```python
from build123d import *

# Parameters (mm, degrees)
SKETCH2_W                   = 29
SKETCH2_H                   = 27.475014389
BOSS_EXTRUDE1_DEPTH         = 2
SKETCH7_W                   = 45
SKETCH7_H                   = 2
BOSS_EXTRUDE2_DEPTH         = 15
TAP_DRILL_FOR_M2X0_4_TAP1_D = 1.6
TAP_DRILL_FOR_M2X0_4_TAP2_D = 1.6


with BuildPart() as part:
    # Sketch2 → Boss-Extrude1 (new body)
    with BuildSketch(Plane(origin=(0, 0, 0), x_dir=(1, 0, 0), z_dir=(0, 1, 0))):
        with Locations((-24.397211382, -13.737507195)):
            Rectangle(SKETCH2_W, SKETCH2_H)
    extrude(amount=BOSS_EXTRUDE1_DEPTH)

    # Sketch7 → Boss-Extrude2 (add)
    with BuildSketch(Plane(origin=(0, 0, 0), x_dir=(-1, 0, 0), z_dir=(0, -1, 0))):
        with Locations((24.397211382, 0.886680676)):
            Rectangle(SKETCH7_W, SKETCH7_H)
    extrude(amount=-BOSS_EXTRUDE2_DEPTH)

    # Tap Drill for M2x0.4 Tap1 (through all)
    with Locations(Plane.XY.offset(0.113319324)):
        with Locations((-42.897211382, 4)):
            Hole(TAP_DRILL_FOR_M2X0_4_TAP1_D / 2)

    # Tap Drill for M2x0.4 Tap2 (through all)
    with Locations(Plane.XY.offset(0.113319324)):
        with Locations((-5.897211382, 4)):
            Hole(TAP_DRILL_FOR_M2X0_4_TAP2_D / 2)


solid = part.part
```
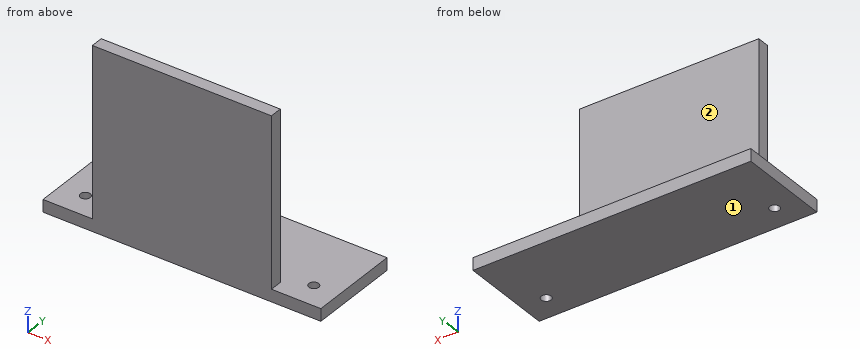
Model file for the job. Use its own axes, mm. Face numbers are marked on the shaded views. A direction names the side the tool comes from. Coordinates: 2 decimals unless noted, no trailing zeros. Loops run counter-clockwise (first coordinate to the right, second up) from the corner with the lowest first, then second, coordinate; pieces in that order, holes last. Notation, with made-up numbers: (16, 83.5) -> (65, 83.5) arc R28 ccw to (65, 120.5) -> close; hole circle Ø6 at (22.5, -17.75). An arc over 180 degrees is marked (long way). Answer as a JSON object with one key per item and string values.
Q1. Flat gauge pins, fed straight in: P1, Ø1, axis at x = -42.9, y = 4, coming from the +Z side; P2, Ø1.6, axis at y = 0.5, z = 7.5, coming from the +X side; P3, Ø4, axis at x = -38.5, z = 13.5, coming from the +Y side; P4, Ø7.5, axis at x = -26, y = 6, coming from the +Z side. Where does each tip first touch, or does it go through?
Report:
{"P1": "passes through", "P2": "stops at x = -9.9", "P3": "stops at y = 2", "P4": "stops at z = 0.11"}
Q2. Cut at A-A (y = 4). List the corners of the cut face in (x, z), and give its area (3 significant figures).
Report:
{"outline": "(-46.9, -1.89) -> (-43.7, -1.89) -> (-43.7, 0.11) -> (-46.9, 0.11) -> close; (-42.1, -1.89) -> (-6.7, -1.89) -> (-6.7, 0.11) -> (-42.1, 0.11) -> close; (-5.1, -1.89) -> (-1.9, -1.89) -> (-1.9, 0.11) -> (-5.1, 0.11) -> close", "area": "83.6 mm2"}
Q3. Cut at D-D (z = 22). List the corners of the cut face in (x, y), and give its area (3 significant figures).
Report:
{"outline": "(-38.9, 0) -> (-9.9, 0) -> (-9.9, 2) -> (-38.9, 2) -> close", "area": "58.0 mm2"}
Q4. Cut at B-B (x = -29.5). List the corners of the cut face in (y, z), and give its area (3 significant figures).
Report:
{"outline": "(0, -1.89) -> (15, -1.89) -> (15, 0.11) -> (2, 0.11) -> (2, 27.48) -> (0, 27.48) -> close", "area": "84.7 mm2"}
Q5. 3-axis set-ups, long thin cutter, end or side, ignore diameter. For the marked faces 1 and 2: which of +Z, -Z, +X, -X, +Y, -Y reach the whole face in a straight line?
Report:
{"face 1": "-Z, +X, -X, +Y, -Y", "face 2": "+Z, +X, -X, +Y"}
Q6. Probe probe 1 along Y at (x, z) = (-26, 19.25); probe 2 along Z at (x, y) = (-4.5, 7.75); probe 3 along X at (y, z) = (1.75, 25.5). List the from-to ranges inside material, lowest first.
Report:
{"probe 1": "y = 0 to 2", "probe 2": "z = -1.89 to 0.11", "probe 3": "x = -38.9 to -9.9"}
Q7. Cut at C-C (y = 12). List the corners of the cut face in (x, z), and give its area (3 significant figures).
Report:
{"outline": "(-46.9, -1.89) -> (-1.9, -1.89) -> (-1.9, 0.11) -> (-46.9, 0.11) -> close", "area": "90.0 mm2"}
